Part model, mm, in its own coordinate system. Coordinates: 2 decimals unless noted, no trailing zeros. Order: outer loops, then holes, each group sorted by start corner. A loop starts at its lowest first (then second) coordinate and runs counter-clockwise, first axis right, second up.
1) Pin check, flat tips, straight feed: pin 1 Ø10 at (x, y) = (14.5, -21.5) entering from +Z; pin 2 Ø11.5 at (x, z) = (20, 1000) entering from +Y. Stop position of each tip, or through.
2) Cut at A-A (y = 16.5). List the corners of the cut face in (x, z).
3) Cut at B-B (z = 1475). List the corners of the cut face in (x, y), and give its area (3 significant figures).
4) Wall check: L1, parallel to X at y = -0.5, z = 1279; L2, parallel to X at y = 29, z = 1600. Give the ranges that are in metal, low to high.
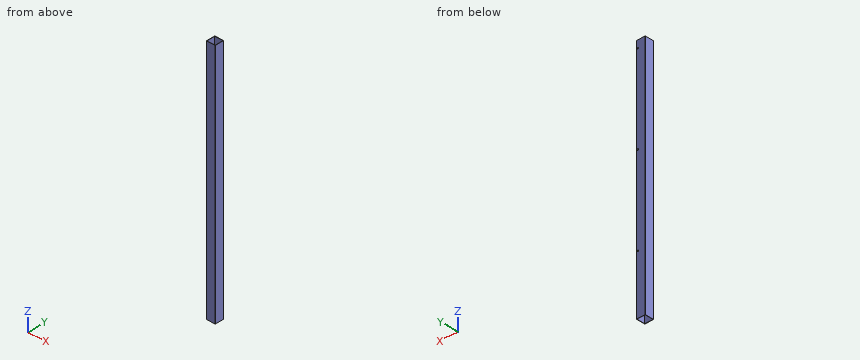
Autodesk Inventor part; units mm, degrees
ref_plane "YZ Plane" through (0, 0, 0) normal (1, 0, 0) x (0, 1, 0)
ref_plane "XZ Plane" through (0, 0, 0) normal (0, 1, 0) x (-1, 0, 0)
ref_plane "XY Plane" through (0, 0, 0) normal (0, 0, 1) x (1, 0, 0)
sketch "Sketch1" plane through (0, 0, 0) normal (0, 0, 1) x (1, 0, 0)
  line L0 (-28, 30) -> (28, 30)
  line L1 (30, 28) -> (30, -28)
  line L2 (28, -30) -> (-28, -30)
  line L3 (-30, -28) -> (-30, 28)
  line L4 (-30, 30) -> (30, -30) construction
  line L5 (28, 28) -> (-28, 28)
  line L6 (-28, 28) -> (-28, -28)
  line L7 (-28, -28) -> (28, -28)
  line L8 (28, -28) -> (28, 28)
  arc A0 (-28, 30) -> (-30, 28) centre (-28, 28) ccw
  arc A1 (30, 28) -> (28, 30) centre (28, 28) ccw
  arc A2 (28, -30) -> (30, -28) centre (28, -28) ccw
  arc A3 (-30, -28) -> (-28, -30) centre (-28, -28) ccw
  point P0 (0, 0)
  point P1 (30, 30)
  point P2 (-30, -30)
  point P3 (0, 0)
  dimension "d0" = 60
  dimension "d1" = 60
  dimension "d2" = 2
  dimension "d3" = 2
extrude "Extrusion1" add sketch "Sketch1" along normal blind 1650
sketch "Sketch2" plane through (-28, 30, 0) normal (0, 1, 0) x (1, 0, 0)
  circle A0 centre (48, -1000) radius 5
  line L0 (56, -1650) -> (0, -1650)
  line L1 (56, 0) -> (0, 0)
  circle A1 centre (48, -400) radius 5
  circle A2 centre (48, -1600) radius 5
  line L2 (48, -116) -> (48, -1518) construction
  line L3 (58, 0) -> (58, -1650)
  point P0 (28, 0)
  dimension "d6" = 10
  dimension "d10" = 1000
  dimension "d11" = 10
  dimension "d12" = 10
  dimension "d13" = 600
  dimension "d14" = 600
  dimension "d15" = 10
extrude "Extrusion2" cut sketch "Sketch2" against normal up to next
properties part number "TABLE_BERAM" material "Stainless Steel"
Geometry check:
1. pin 1: passes through
1. pin 2: stops at y = 30
2. outline: (-30, 0) - (-28, 0) - (-28, 1650) - (-30, 1650) - close; (28, 0) - (30, 0) - (30, 1650) - (28, 1650) - close
3. outline: (-30, -28) arc R2 ccw to (-28, -30) - (28, -30) arc R2 ccw to (30, -28) - (30, 28) arc R2 ccw to (28, 30) - (-28, 30) arc R2 ccw to (-30, 28) - close; hole (-28, -28) - (28, -28) - (28, 28) - (-28, 28) - close
3. area: 461 mm2
4. L1: x = -30 to -28, 28 to 30
4. L2: x = -29.73 to 15, 25 to 29.73
